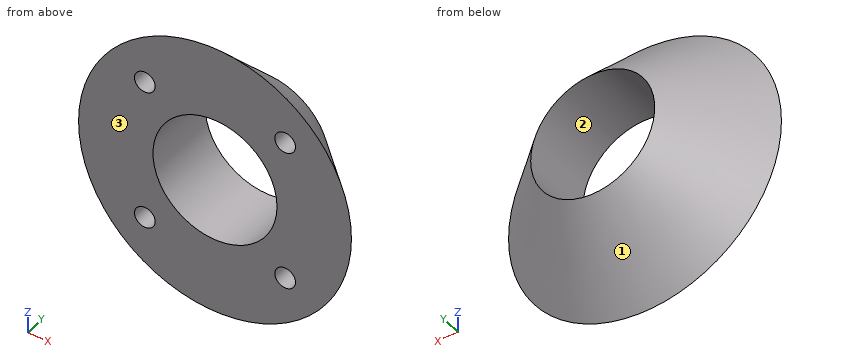
```python
from build123d import *

# Parameters (mm, degrees)
SKETCH001_R  = 1.25
POCKET_DEPTH = 3


with BuildPart() as part:
    # Sketch → Revolution (revolve)
    with BuildSketch(Plane.XY):
        Polygon((7.5, 0), (16.5, 0), (7.5, 9), align=None)
    revolve(axis=Axis((0, 0, 0), (0, 1, 0)))

    # Sketch001 (on Face1 of Revolution) → Pocket (cut)
    with BuildSketch(Plane.XZ):
        with Locations((-8.485281, 8.485281)):
            Circle(SKETCH001_R)
        with Locations((8.485281, 8.485281)):
            Circle(SKETCH001_R)
        with Locations((8.485281, -8.485281)):
            Circle(SKETCH001_R)
        with Locations((-8.485281, -8.485281)):
            Circle(SKETCH001_R)
    extrude(amount=-POCKET_DEPTH, mode=Mode.SUBTRACT)


solid = part.part
```
For this review, take the finished solid that the model builds, in its own axes (mm). Face numbers are marked on the shaded views. Coordinates: 2 decimals unless noted, no trailing zeros. Order: outer loops, then holes, each group sorted by start corner. A loop starts at its lowest first (then second) coordinate and runs counter-clockwise, first axis right, second up. Notation, with made-up numbers: (45.5, 78) - (73.5, 78) arc R17 ccw to (73.5, 95) - close; hole circle Ø8 at (-34.75, 0). An arc over 180 degrees is marked (long way). Answer as a JSON object with one key per item and string values. Group by question number.
1. For probe 1 along Z at (x, y) = (-8, 0.75); probe 2 along Z at (x, y) = (-1.5, 6.75); probe 3 along X at (y, z) = (3, 0.5), list the stretches that pass through material, from the lowest coordinate up.
2. We need section B-B on x = 0. State the section outline as (y, z) points.
3. We need section C-C on y = 8.25. State the section outline as (x, z) points.
4. We need section A-A on z = 0. State the section outline as (x, y) points, then the cut area to 3 significant figures.
5. The part is to be moulded in two halves that separate along Z. For the marked faces 1, 2 and 3, say which applies: pulls with the +Z half, pulls with the -Z half, needs draft (parallel to the pull), parting line crosses it, or undercut.
6. Clearance check with flat-ended pins moving along their axes: P1, Ø2, axis at y = 3, z = -11.5, coming from the -X side; P2, Ø3, axis at x = 8.5, z = -8.5, coming from the -Y side; P3, Ø1, axis at x = 3.5, z = 12.5, coming from the +Y side; P4, Ø3, axis at x = -4, z = -2.5, coming from the -Y side. State where each tip first meets the part, or that it passes through.
7. We need section D-D on y = 4.25. State the section outline as (x, z) points.
Final values:
{
 "1": {"probe 1": "-13.57 to -9.64, -7.33 to 7.33, 9.64 to 13.57", "probe 2": "-9.63 to -7.35, 7.35 to 9.63", "probe 3": "-13.49 to -7.48, 7.48 to 13.49"},
 "2": {"outline": "(0, -16.5) - (9, -7.5) - (0, -7.5) - close; (0, 7.5) - (9, 7.5) - (0, 16.5) - close"},
 "3": {"outline": "circle Ø16.5 at (0, 0); hole circle Ø15 at (0, 0)"},
 "4": {"outline": "(-16.5, 0) - (-7.5, 0) - (-7.5, 9) - close; (7.5, 0) - (16.5, 0) - (7.5, 9) - close", "area": "81.0 mm²"},
 "5": {"face 1": "parting line crosses it", "face 2": "undercut", "face 3": "needs draft"},
 "6": {"P1": "x = -9.26", "P2": "y = 0", "P3": "y = 4.02", "P4": "through"},
 "7": {"outline": "circle Ø24.5 at (0, 0); hole circle Ø15 at (0, 0)"}
}
